Work out the finished part from the listing and answer in its coordinate system (mm). A direction names the side the tool comes from. Coordinates: 2 decimals unless noted, no trailing zeros. Loops run counter-clockwise (first coordinate to the right, second up) from the corner with the lowest first, then second, coordinate; pieces in that order, holes last. Notation, with made-up numbers: (19.25, 0) -> (28.25, 0) arc R21 cw to (28.25, 5) -> close; hole circle Ø3 at (-2, 22.5). An arc over 180 degrees is marked (long way). Answer as CSV lines item,"result".
```python
from build123d import *

# Parameters (mm, degrees)
F1_DEPTH = 3
F2_R     = 1.5
F3_DEPTH = 25
F5_DEPTH = 3


with BuildPart() as f1:
    # F0 (on Front) → F1 (new body)
    with BuildSketch(Plane.XZ):
        with BuildLine():
            Line((-75, -60), (75, -60))
            ThreePointArc((75, -60), (78.535534, -58.535534), (80, -55))
            Line((80, -55), (80, 55))
            ThreePointArc((80, 55), (78.535534, 58.535534), (75, 60))
            Line((75, 60), (-75, 60))
            ThreePointArc((-75, 60), (-78.535534, 58.535534), (-80, 55))
            Line((-80, 55), (-80, -55))
            ThreePointArc((-80, -55), (-78.535534, -58.535534), (-75, -60))
        make_face()
    extrude(amount=F1_DEPTH)

    # F2 (on Front) → F3 (cut)
    with BuildSketch(Plane.XZ):
        with Locations((-75, 55)):
            Circle(F2_R)
        with Locations((75, 55)):
            Circle(F2_R)
        with Locations((75, -55)):
            Circle(F2_R)
        with Locations((-75, -55)):
            Circle(F2_R)
    extrude(amount=F3_DEPTH, mode=Mode.SUBTRACT)

    # F4 (on face) → F5 (cut)
    with BuildSketch(Plane.XZ.offset(3)):
        with BuildLine():
            ThreePointArc((72.5, 48.385622), (71.035534, 51.921156), (67.5, 53.385622))
            Line((67.5, 53.385622), (-67.5, 53.385622))
            ThreePointArc((-67.5, 53.385622), (-71.035534, 51.921156), (-72.5, 48.385622))
            Line((-72.5, 48.385622), (-72.5, -48.385622))
            ThreePointArc((-72.5, -48.385622), (-71.035534, -51.921156), (-67.5, -53.385622))
            Line((-67.5, -53.385622), (67.5, -53.385622))
            ThreePointArc((67.5, -53.385622), (71.035534, -51.921156), (72.5, -48.385622))
            Line((72.5, -48.385622), (72.5, 48.385622))
        make_face()
    extrude(amount=-F5_DEPTH, mode=Mode.SUBTRACT)


solid = f1.part
```
(1) A cutting plane is placed at A-A, the plane z = -29.5. Write down the section's boundary in (x, y).
Computed values:
outline,"(-80, -3) -> (-72.5, -3) -> (-72.5, 0) -> (-80, 0) -> close; (72.5, -3) -> (80, -3) -> (80, 0) -> (72.5, 0) -> close"
(2) A cutting plane is placed at C-C, the plane y = -2.4. Write down the section's boundary in (x, z), and give its area (3 significant figures).
Computed values:
outline,"(-80, -55) arc R5 ccw to (-75, -60) -> (75, -60) arc R5 ccw to (80, -55) -> (80, 55) arc R5 ccw to (75, 60) -> (-75, 60) arc R5 ccw to (-80, 55) -> close; hole circle Ø3 at (-75, -55); hole circle Ø3 at (-75, 55); hole (-72.5, -48.39) arc R5 ccw to (-67.5, -53.39) -> (67.5, -53.39) arc R5 ccw to (72.5, -48.39) -> (72.5, 48.39) arc R5 ccw to (67.5, 53.39) -> (-67.5, 53.39) arc R5 ccw to (-72.5, 48.39) -> close; hole circle Ø3 at (75, -55); hole circle Ø3 at (75, 55)"
area,"3,690 mm2"
(3) For a pull along Z with two mould halves and no side action, classify faces 1 (the face through (-70.996, -1.521, 51.96)), 2 (the face through (0, -3, 54)), 3 (the face through (78, -1, -59)), 4 (the face through (-71.074, -1.521, -51.882)) as pulls with the +Z half, pulls with the -Z half, needs draft (parallel to the pull), parting line crosses it, or undercut.
Computed values:
face 1,"undercut"
face 2,"needs draft"
face 3,"pulls with the -Z half"
face 4,"undercut"
(4) Which of the six approach directions +Z, -Z, +X, -X, +Y, -Y give full straight-line access (tool end or side, diameter ignored) to faces 5 (the face through (70.996, -1.521, -51.96)), 6 (the face through (79, -1, 58))?
Computed values:
face 5,"+Y, -Y"
face 6,"+Z, +X, +Y, -Y"
(5) Consider line 1 along X through (y, z) = (-1.75, 55); line 2 along Z through (x, y) = (75, -1); line 3 along X through (y, z) = (-0.45, 37.5). Determine where each line is inside the solid, lowest interval first.
Computed values:
line 1,"-80 to -76.5, -73.5 to 73.5, 76.5 to 80"
line 2,"-60 to -56.5, -53.5 to 53.5, 56.5 to 60"
line 3,"-80 to -72.5, 72.5 to 80"
(6) A cutting plane is placed at B-B, the plane x = 55. Write down the section's boundary in (y, z).
Computed values:
outline,"(-3, -60) -> (0, -60) -> (0, -53.39) -> (-3, -53.39) -> close; (-3, 53.39) -> (0, 53.39) -> (0, 60) -> (-3, 60) -> close"
